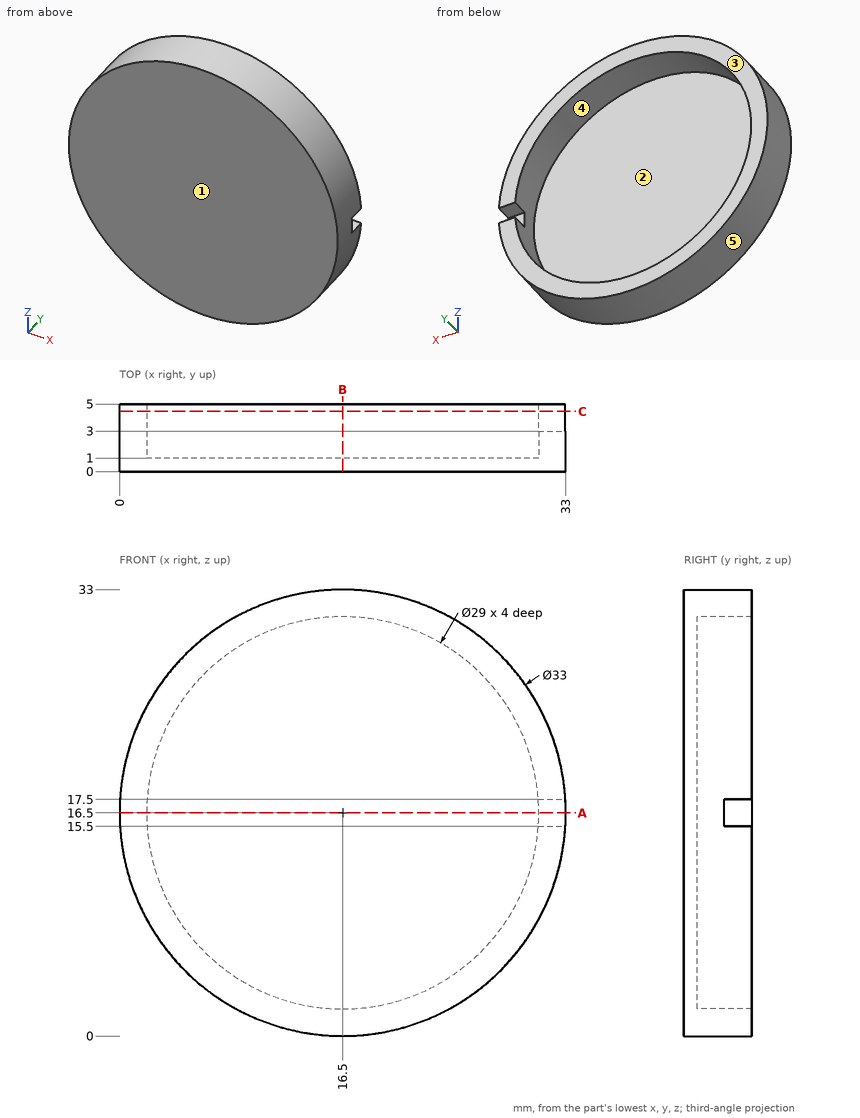
Could you check a few things on this drawing? It's one solid part, dimensions in mm from its lowest x, y, z. A direction names the side the tool comes from. Round coordinates to 2 decimals unless told otherwise and drop trailing zeros. Write each loop counter-clockwise with the first axis right and the second up, starting at its lowest first coordinate (ties: lowest second). Pieces come first, ordered by that corner, then holes. Notation, with made-up numbers: (37.25, -3) -> (89.25, -3) arc R23 cw to (89.25, 10) -> close; hole circle Ø7 at (54, 12.25). An arc over 180 degrees is marked (long way). Use a Markdown table: item, result.
1. Please list where these lines run through material, in increasing order: probe 1 along X at (y, z) = (2, 16.5); probe 2 along Y at (x, z) = (12, 7.5).
Answer key:
| item | result |
|---|---|
| probe 1 | x = 0 to 2, 31 to 33 |
| probe 2 | y = 0 to 1 |
2. We'd pull the mould along X, two halves only. Please class the marked faces 3, 4 and 5: +X half, -X half, draft (parallel to the pull), parting line (faces both ways), or undercut.
Answer key:
| item | result |
|---|---|
| face 3 | draft |
| face 4 | undercut |
| face 5 | parting line |
3. If we section it at B-B (x = 16.5): List the corners of the cut face in (y, z) for me.
Answer key:
| item | result |
|---|---|
| outline | (0, 0) -> (5, 0) -> (5, 2) -> (1, 2) -> (1, 31) -> (5, 31) -> (5, 33) -> (0, 33) -> close |
4. If we section it at C-C (y = 4.45): List the corners of the cut face in (x, z) for me, then the cut area to 3 significant figures.
Answer key:
| item | result |
|---|---|
| outline | (30.97, 15.5) arc R14.5 cw (long way) to (30.97, 17.5) -> (32.97, 17.5) arc R16.5 ccw (long way) to (32.97, 15.5) -> close |
| area | 191 mm^2 |
5. Which directions (+Z, -Z, +X, -X, +Y, -Y) give clear straight access to the entire face, cutting with the end or side of a thin tool? Please do the marked faces 1 and 2.
Answer key:
| item | result |
|---|---|
| face 1 | +Z, -Z, +X, -X, -Y |
| face 2 | +Y |
6. If we section it at A-A (z = 16.5): List the corners of the cut face in (x, y) for me.
Answer key:
| item | result |
|---|---|
| outline | (0, 0) -> (33, 0) -> (33, 3) -> (31, 3) -> (31, 1) -> (2, 1) -> (2, 5) -> (0, 5) -> close |
7. For pin 1 Ø3 at (y, z) = (1.5, 29.5) entering from +X; pin 2 Ø4 at (x, z) = (18.5, 27) entering from +Y; pin 3 Ø1.6 at (x, y) = (32, 4) entering from +Z; pin 4 Ø6 at (x, z) = (13, 13.5) entering from -Y, each with a flat end and sliding along its axis, tell me the tip position at first contact or that it passes through.
Answer key:
| item | result |
|---|---|
| pin 1 | stops at x = 28.33 |
| pin 2 | stops at y = 1 |
| pin 3 | stops at z = 23.99 |
| pin 4 | stops at y = 0 |
